```python
from build123d import *

# Parameters (mm, degrees)
SKETCH1_W           = 150
SKETCH1_H           = 75
BOSS_EXTRUDE1_DEPTH = 60
SKETCH2_R           = 20
BOSS_EXTRUDE2_DEPTH = 60
BOSS_EXTRUDE3_DEPTH = 20


with BuildPart() as part:
    # Sketch1 → Boss-Extrude1 (new body)
    with BuildSketch(Plane(origin=(0, 0, 0), x_dir=(1, 0, 0), z_dir=(0, 1, 0))):
        Rectangle(SKETCH1_W, SKETCH1_H)
    extrude(amount=BOSS_EXTRUDE1_DEPTH)

    # Sketch2 → Boss-Extrude2 (add)
    with BuildSketch(Plane(origin=(0, 60, 0), x_dir=(1, 0, 0), z_dir=(0, 1, 0))):
        with Locations(Location((0, 0, 0), (0, 0, 270))):
            Circle(SKETCH2_R)
    extrude(amount=BOSS_EXTRUDE2_DEPTH)

    # Sketch3 → Boss-Extrude3 (add)
    with BuildSketch(Plane.XY.offset(37.5)):
        with BuildLine():
            Line((-20.750294914, 47.150331809), (22.895664326, 47.150331809))
            ThreePointArc((22.895664326, 47.150331809), (29.966732138, 44.221399621), (32.895664326, 37.150331809))
            Line((32.895664326, 37.150331809), (32.895664326, 27.472721601))
            ThreePointArc((32.895664326, 27.472721601), (29.966732138, 20.401653789), (22.895664326, 17.472721601))
            Line((22.895664326, 17.472721601), (-20.750294914, 17.472721601))
            ThreePointArc((-20.750294914, 17.472721601), (-27.821362726, 20.401653789), (-30.750294914, 27.472721601))
            Line((-30.750294914, 27.472721601), (-30.750294914, 37.150331809))
            ThreePointArc((-30.750294914, 37.150331809), (-27.821362726, 44.221399621), (-20.750294914, 47.150331809))
        make_face()
    extrude(amount=BOSS_EXTRUDE3_DEPTH)


solid = part.part
```
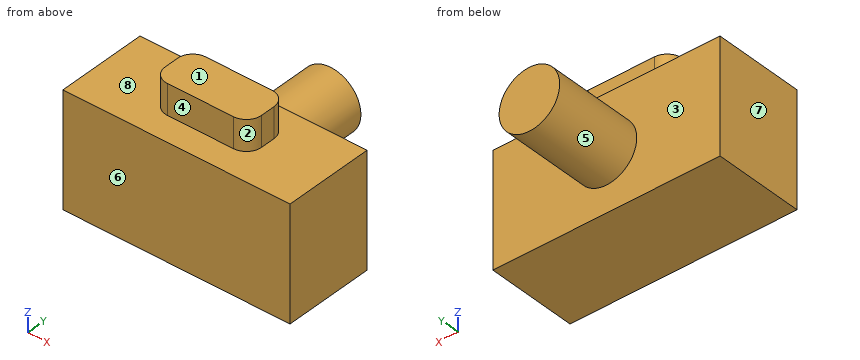
Design review of the part built by this model. Coordinates are the model's own, in mm. Face numbers are marked on the shaded views. A direction names the side the tool comes from. Round coordinates to 2 decimals unless told otherwise and drop trailing zeros. Write each loop counter-clockwise with the first axis right and the second up, starting at its lowest first coordinate (ties: lowest second). Pieces come first, ordered by that corner, then holes.
Item 1: We need section B-B on z = 0. Write out the cut boundary in (x, y), and give its area (3 significant figures).
Item 2: The part is to be moulded in two halves that separate along Y. For the marked faces 1, 2 and 3, say which applies: +Y half, -Y half, draft (parallel to the pull), parting line (faces both ways), or undercut.
Item 3: For probe 1 along Z at (x, y) = (-68, 18); probe 2 along Y at (x, z) = (-19, 9); probe 3 along Y at (x, z) = (-0.5, 42.5), list the stretches that pass through material, from the lowest coordinate up.
Item 4: We need section C-C on y = 83.5. Write out the cut boundary in (x, z), and give its area (3 significant figures).
Item 5: Clearance check with flat-ended pins moving along their axes: pin 1 Ø3 at (y, z) = (32.5, 43) entering from -X; pin 2 Ø12 at (y, z) = (68.5, 44) entering from +X; pin 3 Ø5 at (x, y) = (-40.5, 52.5) entering from +Z; pin 4 Ø22 at (x, z) = (2, 52) entering from +Y. State where each tip first meets the part, or that it passes through.
Item 6: We need section D-D on z = 50.5. Write out the cut boundary in (x, y), and give its area (3 significant figures).
Item 7: For the marked faces 4, 5, 6, 7 and 8, list the 3-axis set-ups (+Z, -Z, +X, -X, +Y, -Y) from which the entire face can be reached by the end or side of a thin tool; tool diameter is ignored.
Item 8: We need section A-A on x = 0. Write out the cut boundary in (y, z).
Returned:
1. outline: (-75, 0) - (75, 0) - (75, 60) - (20, 60) - (20, 120) - (-20, 120) - (-20, 60) - (-75, 60) - close
1. area: 11,400 mm2
2. face 1: draft
2. face 2: -Y half
2. face 3: +Y half
3. probe 1: z = -37.5 to 37.5
3. probe 2: y = 0 to 60
3. probe 3: y = 17.47 to 47.15
4. outline: circle Ø40 at (0, 0)
4. area: 1,260 mm2
5. pin 1: stops at x = -30.75
5. pin 2: passes through
5. pin 3: stops at z = 37.5
5. pin 4: stops at y = 47.15
6. outline: (-30.75, 27.47) arc R10 ccw to (-20.75, 17.47) - (22.9, 17.47) arc R10 ccw to (32.9, 27.47) - (32.9, 37.15) arc R10 ccw to (22.9, 47.15) - (-20.75, 47.15) arc R10 ccw to (-30.75, 37.15) - close
6. area: 1,800 mm2
7. face 4: +Z, +X, -X, -Y
7. face 5: +Y
7. face 6: +Z, -Z, +X, -X, -Y
7. face 7: +Z, -Z, -X, +Y, -Y
7. face 8: +Z
8. outline: (0, -37.5) - (60, -37.5) - (60, -20) - (120, -20) - (120, 20) - (60, 20) - (60, 37.5) - (47.15, 37.5) - (47.15, 57.5) - (17.47, 57.5) - (17.47, 37.5) - (0, 37.5) - close
